```python
from build123d import *

# Parameters (mm, degrees)
F2_R    = 5.08
F3_SIZE = 5.08


# Not quite as in the source:
# - the program builds the solid bodies; features that only make, move or delete a surface that nothing else refers to are left out


with BuildPart() as f1:
    # F0 (on Front) → F1 (revolve)
    with BuildSketch(Plane.XZ):
        Polygon((18.1504152715, 44.5240847766), (0, 44.5240847766), (0, 14.0017503873), (41.8570823967, 14.0017503873), (41.8570823967, 25.5587510765), (18.1504152715, 25.5587510765), align=None)
    revolve(axis=Axis((21.6693747789, 0, 0), (1, 0, 0)))

    # F2
    f2_edges = [f1.edges().sort_by_distance(p)[0] for p in [
        (18.150415, 0, -25.558751),
    ]]
    fillet(f2_edges, radius=F2_R)

    # F3
    f3_edges = [f1.edges().sort_by_distance(p)[0] for p in [
        (41.857082, 0, -25.558751),
        (18.150415, 0, -44.524085),
        (0, 0, -44.524085),
    ]]
    chamfer(f3_edges, length=F3_SIZE)


solid = f1.part
```
The model under review builds one solid part; all positions refer to its coordinate system, in mm. A direction names the side the tool comes from. Round coordinates to 2 decimals unless told otherwise and drop trailing zeros. Loops run counter-clockwise (first coordinate to the right, second up) from the corner with the lowest first, then second, coordinate; pieces in that order, holes last. Notation, with made-up numbers: (-28.75, 81) - (21.25, 81) arc R5 ccw to (21.25, 86) - close; hole circle Ø7 at (-31.75, -22). An arc over 180 degrees is marked (long way). Use a Markdown table: item, result. Add a question column.
Q1. Insertion check: pin 1 Ø1.5 at (y, z) = (14, 33) entering from -X; pin 2 Ø2 at (x, y) = (17, 32.5) entering from +Z; pin 3 Ø3 at (y, z) = (23.5, 5.5) entering from +X; pin 4 Ø3 at (y, z) = (-26.5, 27) entering from +X. Each pin has a flat end and moves straight along its axis. Give the tip position at first contact, or say it passes through.
Q2. Add section A-A (y = 0). State the section outline as (x, z) points, plus the area to 3 significant figures.
Q3. Add section C-C (x = 11.5). State the section outline as (y, z) points, plus the area to 3 significant figures.
Q4. For probe 1 along Y at (x, z) = (24, 0); probe 2 along X at (y, z) = (-29, -24); probe 3 along Z at (x, y) = (22, 0), list the stretches that pass through material, from the lowest coordinate up.
Q5. Machinability: for faces 1 (the face through (29.91, 24.95, -5.54)), 2 (the face through (0.2, 38.7, -8.6)), which of the approach directions +Z, -Z, +X, -X, +Y, -Y give a long, thin tool a straight path to every point of the face, cutting with its end or side? Answer none if there is none.
Q6. Add section D-D (x = 33.5). State the section outline as (y, z) points, plus the area to 3 significant figures.
Worked answers:
| question | item | result |
|---|---|---|
| 1 | pin 1 | x = 0 |
| 1 | pin 2 | z = 26.38 |
| 1 | pin 3 | x = 39.7 |
| 1 | pin 4 | x = 18.15 |
| 2 | outline | (0, -39.44) - (5.08, -44.52) - (13.07, -44.52) - (18.15, -39.44) - (18.15, -30.64) arc R5.08 cw to (23.23, -25.56) - (36.78, -25.56) - (41.86, -20.48) - (41.86, -14) - (0, -14) - close; (0, 14) - (41.86, 14) - (41.86, 20.48) - (36.78, 25.56) - (23.23, 25.56) arc R5.08 cw to (18.15, 30.64) - (18.15, 39.44) - (13.07, 44.52) - (5.08, 44.52) - (0, 39.44) - close |
| 2 | area | 1,590 mm² |
| 3 | outline | circle Ø89.05 at (0, 0); hole circle Ø28 at (0, 0) |
| 3 | area | 5,610 mm² |
| 4 | probe 1 | -25.56 to -14, 14 to 25.56 |
| 4 | probe 2 | 0 to 18.15 |
| 4 | probe 3 | -25.71 to -14, 14 to 25.71 |
| 5 | face 1 | +X |
| 5 | face 2 | -X |
| 6 | outline | circle Ø51.12 at (0, 0); hole circle Ø28 at (0, 0) |
| 6 | area | 1,440 mm² |
